Autodesk Inventor part; units mm, degrees
ref_plane "YZ Plane" through (0, 0, 0) normal (1, 0, 0) x (0, 1, 0)
ref_plane "XZ Plane" through (0, 0, 0) normal (0, 1, 0) x (-1, 0, 0)
ref_plane "XY Plane" through (0, 0, 0) normal (0, 0, 1) x (1, 0, 0)
sketch "Sketch1" plane through (0, 0, 0) normal (0, 1, 0) x (-1, 0, 0)
  line L0 (65, 65) -> (-65, 65)
  line L1 (-65, 65) -> (-65, -65)
  line L2 (-65, -65) -> (65, -65)
  line L3 (65, -65) -> (65, 65)
  line L4 (65, 65) -> (-65, -65) construction
  line L5 (-65, 65) -> (65, -65) construction
  point P0 (0, 0)
  dimension "d0" = 130
  dimension "d1" = 130
extrude "Extrusion1" add sketch "Sketch1" along normal blind 30
shell "Shell1" thickness 3 removed faces 1 at (21.6667, 30, -21.6667)
sketch "Sketch2" plane through (-62, 3, -62) normal (0, 1, 0) x (1, 0, 0)
  line L0 (129.611, -53.7228) -> (-3, -53.7228)
  line L1 (-3, -53.7228) -> (-3, -70.2772)
  line L2 (-3, -70.2772) -> (129.611, -70.2772)
  line L3 (129.611, -70.2772) -> (129.611, -53.7228)
  line L4 (53.8994, 0) -> (53.8994, -127.3663)
  line L5 (53.8994, -127.3663) -> (70.1006, -127.3663)
  line L6 (70.1006, -127.3663) -> (70.1006, 0)
  line L7 (70.1006, 0) -> (53.8994, 0)
  line L8 (0, 0) -> (124, 0)
  line L9 (-3, 3) -> (-3, -127)
  line L10 (124, -124) -> (124, 0)
  line L11 (124, 0) -> (0, 0)
  line L12 (0, 0) -> (0, -124)
  line L13 (0, -124) -> (124, -124)
  point P0 (62, -62)
  point P1 (63.6106, -64.6568)
  point P2 (62, 0)
  point P3 (-3, -62)
  point P4 (70.1006, -124)
  point P5 (124, -70.2772)
  point P6 (70.1006, -70.2772)
  point P7 (124, -53.7228)
  point P8 (70.1006, 0)
  point P9 (70.1006, -53.7228)
  point P10 (0, -53.7228)
  point P11 (53.8994, -53.7228)
  point P12 (53.8994, 0)
  point P13 (53.8994, -124)
  point P14 (53.8994, -70.2772)
  point P15 (0, -70.2772)
  dimension "d5" = 16.5545
  dimension "d6" = 16.2012
extrude "Extrusion2" cut sketch "Sketch2" against normal through all contours L0 L6 L8 L10 | L10 L13 L6 L2 | L0 L12 L8 L4 | L4 L13 L12 L2
sketch "Sketch3" plane through (-65, 0, 65) normal (0, 0, 1) x (1, 0, 0)
  line L0 (3, 27) -> (127, 27)
  line L1 (127, 27) -> (127, 5)
  line L2 (127, 5) -> (3, 5)
  line L3 (3, 5) -> (3, 27)
  line L4 (3, 27) -> (127, 5) construction
  line L5 (127, 27) -> (3, 5) construction
  line L6 (0, 0) -> (130, 0)
  line L7 (0, 0) -> (0, 30)
  line L8 (130, 0) -> (130, 30)
  line L9 (0, 30) -> (130, 30)
  point P0 (65, 0)
  point P1 (65, 16)
  dimension "d9" = 5
  dimension "d10" = 3
  dimension "d11" = 3
  dimension "d12" = 3
extrude "Extrusion3" cut sketch "Sketch3" against normal blind 25.4 contours L0 L1 L2 L3
sketch "Sketch4" plane through (-62, 3, 65) normal (0, 1, 0) x (1, 0, 0)
  circle A0 centre (62, 65) radius 6
  dimension "d15" = 12
extrude "Extrusion4" cut sketch "Sketch4" against normal blind 25.4
pattern_circular "Circular Pattern1" count 4 over 360 about axis through (0, 3, 0) along (0, -1, 0) of "Extrusion3"
properties part number "Ground Support (Topologi)"
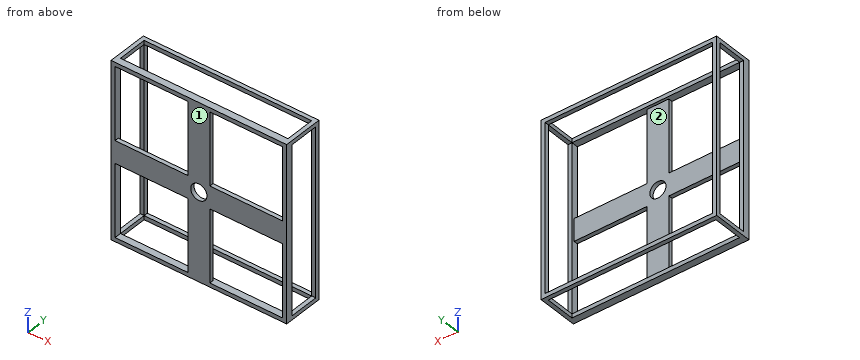
Input: part model. Units: mm. Frame: model coordinates. Face numbers are marked on the shaded views. Give positions to 0.01 mm unless a question says otherwise; leave off trailing zeros. Order: outer loops, then holes, each group sorted by start corner. A loop starts at its lowest first (then second) coordinate and runs counter-clockwise, first axis right, second up. Notation, with made-up numbers: (24, 25.25) - (32, 25.25) arc R34 ccw to (32, 60.25) - close; hole circle Ø6 at (69.25, 9.25). An arc over 180 degrees is marked (long way). Answer as a JSON object with one key per item and string values. Group by question number.
Q1. Cut plane A-A, the plane x = 0. Output: boundary loops of the cut face in (y, z).
Q2. Cut plane D-D, the plane x = -34.5. Output: boundary loops of the cut face in (y, z).
Q3. Cut plane C-C, the plane z = 12. Output: boundary loops of the cut face in (x, y).
Q4. Line query: probe 1 along X at (y, z) = (2.05, 0); probe 2 along Z at (x, y) = (-9.5, 27.75). Output: solid intervals per line, ascending.
Q5. Mould query, pull axis X, two halves, no side actions, for the marked faces 1 and 2. Classes: pulls with the +X half, pulls with the -X half, needs draft (parallel to the pull), parting line crosses it, or undercut.
Q6. Cut plane B-B, the plane y = 17.5. Output: boundary loops of the cut face in (x, z), then the cut area to 3 significant figures.
Results:
{
 "1": {"outline": "(0, -65) - (5, -65) - (5, -62) - (3, -62) - (3, -6) - (0, -6) - close; (0, 6) - (3, 6) - (3, 62) - (5, 62) - (5, 65) - (0, 65) - close; (27, -65) - (30, -65) - (30, -62) - (27, -62) - close; (27, 62) - (30, 62) - (30, 65) - (27, 65) - close"},
 "2": {"outline": "(0, -65) - (5, -65) - (5, -62) - (0, -62) - close; (0, -8.28) - (3, -8.28) - (3, 8.28) - (0, 8.28) - close; (0, 62) - (5, 62) - (5, 65) - (0, 65) - close; (27, -65) - (30, -65) - (30, -62) - (27, -62) - close; (27, 62) - (30, 62) - (30, 65) - (27, 65) - close"},
 "3": {"outline": "(-65, 0) - (-62, 0) - (-62, 5) - (-65, 5) - close; (-65, 27) - (-62, 27) - (-62, 30) - (-65, 30) - close; (-8.1, 0) - (8.1, 0) - (8.1, 3) - (-8.1, 3) - close; (62, 0) - (65, 0) - (65, 5) - (62, 5) - close; (62, 27) - (65, 27) - (65, 30) - (62, 30) - close"},
 "4": {"probe 1": "-65 to -6, 6 to 65", "probe 2": "-65 to -62, 62 to 65"},
 "5": {"face 1": "needs draft", "face 2": "undercut"},
 "6": {"outline": "(-65, -65) - (-62, -65) - (-62, -62) - (-65, -62) - close; (-65, 62) - (-62, 62) - (-62, 65) - (-65, 65) - close; (62, -65) - (65, -65) - (65, -62) - (62, -62) - close; (62, 62) - (65, 62) - (65, 65) - (62, 65) - close", "area": "36.0 mm^2"}
}
